Autodesk Inventor part; units mm, degrees
ref_plane "YZ Plane" through (0, 0, 0) normal (1, 0, 0) x (0, 1, 0)
ref_plane "XZ Plane" through (0, 0, 0) normal (0, 1, 0) x (-1, 0, 0)
ref_plane "XY Plane" through (0, 0, 0) normal (0, 0, 1) x (1, 0, 0)
sketch "Sketch1" plane through (0, 0, 0) normal (0, 0, 1) x (1, 0, 0)
  line L0 (0, 0) -> (-28.575, 0)
  line L1 (-28.575, 0) -> (-28.575, 19.05)
  line L2 (-28.575, 19.05) -> (0, 19.05)
  line L3 (0, 19.05) -> (0, 0)
  line L4 (-14.2875, 0) -> (-14.2875, 6.35)
  circle A0 centre (-14.2875, 6.35) radius 2.3812
  dimension "d0" = 28.575
  dimension "d1" = 19.05
  dimension "d2" = 6.35
  dimension "d3" = 4.7625
extrude "Plate1" add sketch "Sketch1" along normal blind 3.175
sketch "Sketch5" plane through (0, 28.575, -9.525) normal (0, 1, 0) x (-1, 0, 0)
  line L0 (28.575, 0) -> (0, 0)
  line L1 (0, 0) -> (0, -12.7)
  line L2 (0, -12.7) -> (28.575, -12.7)
  line L3 (28.575, -12.7) -> (28.575, 0)
edge flange "Flange3" height 25.4 angle 90 thickness 3.175 bend radius 9.525 thickness toward (0, 1, 0) relief tear relief width 3.175 relief depth 1.5875 edges at (-14.2875, 19.05, 0) wall of the first edge with corners at (-28.575, 28.575, -9.525) (0, 28.575, -9.525) (0, 28.575, -22.225) (-28.575, 28.575, -22.225)
bend "Bend3"
corner "Corner3"
sketch "Sketch6" plane through (0, 19.05, -31.75) normal (0, 0, -1) x (-1, 0, 0)
  line L0 (28.575, 0) -> (0, 0)
  line L1 (0, 0) -> (0, -19.05)
  line L2 (0, -19.05) -> (28.575, -19.05)
  line L3 (28.575, -19.05) -> (28.575, 0)
edge flange "Flange4" height 31.75 angle 90 thickness 3.175 bend radius 9.525 thickness toward (0, 0, -1) relief tear relief width 3.175 relief depth 1.5875 edges at (-14.2875, 28.575, -22.225) wall of the first edge with corners at (-28.575, 19.05, -31.75) (0, 19.05, -31.75) (0, 0, -31.75) (-28.575, 0, -31.75)
bend "Bend4"
corner "Corner4"
sketch "Sketch7" plane through (0, 0, -34.925) normal (0, 0, -1) x (-1, 0, 0)
  circle A0 centre (14.2875, 6.35) radius 2.3812
  circle A1 centre (14.2875, 6.35) radius 2.3812
extrude "Cut2" cut sketch "Sketch7" against normal blind 3.175
sketch "Sketch8" plane through (-28.575, 31.75, -9.525) normal (0, 1, 0) x (1, 0, 0)
  line L0 (28.575, 12.7) -> (28.575, 0)
  line L1 (0, 0) -> (0, 12.7)
  line L2 (0, 5.8436) -> (6.35, 5.8436)
  circle A0 centre (6.35, 5.8436) radius 3.3782
  line L3 (28.575, 5.8436) -> (22.225, 5.8436)
  circle A1 centre (22.225, 5.8436) radius 3.3782
  point P0 (28.575, -9.525)
  dimension "d51" = 6.35
  dimension "d52" = 6.7564
  dimension "d53" = 6.35
  dimension "d54" = 6.7564
extrude "Cut3" cut sketch "Sketch8" against normal blind 3.175
sketch "Sketch9" plane through (-28.575, 31.75, -9.525) normal (0, 1, 0) x (1, 0, 0)
  circle A0 centre (6.35, 5.8436) radius 3.3782
  circle A1 centre (22.225, 5.8436) radius 3.3782
  line L0 (0, 0) -> (28.575, 0)
  line L1 (28.575, 12.7) -> (28.575, 0)
  line L2 (0, 12.7) -> (28.575, 12.7)
  line L3 (0, 0) -> (0, 12.7)
  point P0 (28.575, -9.525)
sketch "Sketch10" plane through (-28.575, 28.575, -9.525) normal (0, -1, 0) x (1, 0, 0)
  circle A0 centre (6.35, -5.8436) radius 3.3782
  circle A1 centre (22.225, -5.8436) radius 3.3782
  line L0 (28.575, 0) -> (0, 0)
  line L1 (0, -12.7) -> (0, 0)
  line L2 (0, -12.7) -> (28.575, -12.7)
  line L3 (28.575, -12.7) -> (28.575, 0)
  point P0 (28.575, 9.525)
equation "\"d49\" = Thickness"
equation "\"d55\" = Thickness"
equation "\"d29\" = BendReliefWidth"
equation "\"d30\" = BendReliefDepth"
equation "\"d31\" = MinimumRemnant"
equation "\"d32\" = BendRadius"
equation "\"d36\" = CornerReliefSize"
equation "\"d37\" = GapSize"
equation "\"d38\" = JacobiRadiusSize"
equation "\"d39\" = BendReliefWidth"
equation "\"d40\" = BendReliefDepth"
equation "\"d41\" = MinimumRemnant"
equation "\"d42\" = BendRadius"
equation "\"d46\" = CornerReliefSize"
equation "\"d47\" = GapSize"
equation "\"d48\" = JacobiRadiusSize"
equation "\"BendRadius\" = Thickness"
equation "\"BendReliefWidth\" = Thickness"
equation "\"BendReliefDepth\" = 0.5 * Thickness"
equation "\"CornerReliefSize\" = 4 * Thickness"
equation "\"MinimumRemnant\" = 2 * Thickness"
equation "\"TransitionRadius\" = BendRadius"
equation "\"JacobiRadiusSize\" = BendRadius"
equation "\"GapSize\" = Thickness"
equation "\"d4\" = BendRadius"
properties part number "pulley mount" material "Aluminum 6061"
For this review, take the finished solid that the model builds, in its own axes (mm). A direction names the side the tool comes from. Round coordinates to 2 decimals unless told otherwise and drop trailing zeros. Order: outer loops, then holes, each group sorted by start corner. A loop starts at its lowest first (then second) coordinate and runs counter-clockwise, first axis right, second up. Notation, with made-up numbers: M 27.25,73 L 60.25,73 A17 cw 60.25,87 Z; hole C -37.5,-36 d8. An arc over 180 degrees is marked long. Use a Markdown table: item, result. Add a question column.
Item 1: Add section D-D, the plane y = 11. Give the boundary of the cut face in (x, z) (3 decimals), then the cut area to 3 significant figures.
Item 2: Add section A-A, the plane y = 6.35. Give the boundary of the cut face in (x, z) (3 decimals), then the cut area to 3 significant figures.
Item 3: To check wall thickness, follow line 1 along Z through (x, y) = (-18.5, 14) (3 decimals); line 2 along Z through (x, y) = (-23.5, 19.5); line 3 along X through (y, z) = (6.35, 1.1) (3 decimals). State the ranges of each line that lie inside material, in increasing order.
Item 4: Add section C-C, the plane z = -17.5. Give the boundary of the cut face in (x, y) (3 decimals), then the cut area to 3 significant figures.
Item 5: Mouldability with a two-part tool opening along Z and no side actions: class faces 3 (the flat face through (-14, 10, -31.75)), 4 (the flat face through (-14, 31.75, -16)), 5 (the cylindrical face through (-22.66, 30.18, -18.72)), 6 (the cylindrical face through (-14.087, 27.931, -31.303)) as released by +Z, released by -Z, zero draft, split by the parting line, or undercut.
Item 6: Tool access review of faces 1 (the flat face through (-14, 28.575, -16)), 2 (the cylindrical face through (-11.91, 6.45, -33.36)): name each direction out of +Z, -Z, +X, -X, +Y, -Y from which nothing blocks a thin tool from reaching the whole face with its end or side.
Item 7: Insertion check: pin 1 (11 mm diameter, centred on x = -6.35, z = -15.37, fed in from -Y) (3 decimals); pin 2 (5 mm diameter, centred on x = -5.5, z = -2, fed in from +Y); pin 3 (14 mm diameter, centred on x = -10.5, z = -13, fed in from -Y); pin 4 (3 mm diameter, centred on x = -14.29, y = 6.35, fed in from +Z). Each pin has a flat end and moves straight along its axis. Give the tip position at first contact, or say it passes through.
Item 8: Add section B-B, the plane x = -6.35. Give the boundary of the cut face in (y, z) (3 decimals), then the cut area to 3 significant figures.
Geometry results:
| question | item | result |
|---|---|---|
| 1 | outline | M -28.575,-34.925 L 0,-34.925 L 0,-31.75 L -28.575,-31.75 Z; M -28.575,0 L 0,0 L 0,3.175 L -28.575,3.175 Z |
| 1 | area | 181 mm² |
| 2 | outline | M -28.575,-34.925 L -16.669,-34.925 L -16.669,-31.75 L -28.575,-31.75 Z; M -28.575,0 L -16.669,0 L -16.669,3.175 L -28.575,3.175 Z; M -11.906,-34.925 L 0,-34.925 L 0,-31.75 L -11.906,-31.75 Z; M -11.906,0 L 0,0 L 0,3.175 L -11.906,3.175 Z |
| 2 | area | 151 mm² |
| 3 | line 1 | z = -34.925 to -31.75, 0 to 3.175 |
| 3 | line 2 | z = -34.92 to -31.74, -0.01 to 3.17 |
| 3 | line 3 | x = -28.575 to -16.669, -11.906 to 0 |
| 4 | outline | M -28.575,28.575 L -24.846,28.575 L -24.846,31.75 L -28.575,31.75 Z; M -19.604,28.575 L -8.971,28.575 L -8.971,31.75 L -19.604,31.75 Z; M -3.729,28.575 L 0,28.575 L 0,31.75 L -3.729,31.75 Z |
| 4 | area | 57.4 mm² |
| 5 | face 3 | undercut |
| 5 | face 4 | zero draft |
| 5 | face 5 | undercut |
| 5 | face 6 | released by -Z |
| 6 | face 1 | +X, -X, -Y |
| 6 | face 2 | +Z, -Z |
| 7 | pin 1 | stops at y = 28.575 |
| 7 | pin 2 | stops at y = 30.71 |
| 7 | pin 3 | stops at y = 27.9 |
| 7 | pin 4 | passes through |
| 8 | outline | M 0,-34.925 L 19.05,-34.925 A12.7 ccw 31.75,-22.225 L 31.75,-18.747 L 28.575,-18.747 L 28.575,-22.225 A9.525 cw 19.05,-31.75 L 0,-31.75 Z; M 0,0 L 19.05,0 A9.525 cw 28.575,-9.525 L 28.575,-11.99 L 31.75,-11.99 L 31.75,-9.525 A12.7 ccw 19.05,3.175 L 0,3.175 Z |
| 8 | area | 251 mm² |
